Check sheet for the modelled part. Datum: model origin and axes. Units: mm. Round coordinates to 2 decimals unless told otherwise and drop trailing zeros. Write each loop counter-clockwise with the first axis right and the second up, starting at its lowest first coordinate (ties: lowest second). Pieces come first, ordered by that corner, then holes. Notation, with made-up numbers: (10.25, 19.5) -> (17.25, 19.5) arc R14 cw to (17.25, 41.5) -> close; hole circle Ø7 at (56.5, 8). An arc over 180 degrees is marked (long way). One line per item, written item: value.
from build123d import *

# Parameters (mm, degrees)
F1_DEPTH = 10
F3_DEPTH = 35
F5_DEPTH = 45.001


with BuildPart() as f1:
    # F0 (on Right) → F1 (new body)
    with BuildSketch(Plane.YZ):
        with BuildLine():
            ThreePointArc((0, 0), (-34.0398401022, -11.614694955), (-68.0796802044, 0))
            ThreePointArc((-68.0796802044, 0), (-43.0772294723, -14.2909034111), (-14.4906720078, -10.8036128804))
            ThreePointArc((-14.4906720078, -10.8036128804), (-6.7062533875, -6.1248672779), (0, 0))
        make_face()
        with BuildLine():
            ThreePointArc((0, 0), (-6.7062533875, -6.1248672779), (-14.4906720078, -10.8036128804))
            Line((-14.4906720078, -10.8036128804), (0, -10.8036128804))
            Line((0, -10.8036128804), (0, 0))
        make_face()
    extrude(amount=F1_DEPTH)

    # F2 (on face) → F3 (join)
    with BuildSketch(Plane(origin=(0, 0, 0), x_dir=(0, -1, 0), z_dir=(-1, 0, 0))):
        with BuildLine():
            Line((0, -10.8036128804), (14.4906720078, -10.8036128804))
            Line((14.4906720078, -10.8036128804), (14.4906720078, -8.0706065552))
            ThreePointArc((14.4906720078, -8.0706065552), (6.9431775325, -4.5778249918), (0, 0))
            Line((0, 0), (0, -10.8036128804))
        make_face()
    extrude(amount=F3_DEPTH)

    # F4 (on face) → F5 (cut, through all)
    with BuildSketch(Plane.YZ.offset(10)):
        with BuildLine():
            Line((-14.4906720078, -8.0706065552), (-14.4906720078, -10.8036128804))
            Line((-14.4906720078, -10.8036128804), (0, -10.8036128804))
            Line((0, -10.8036128804), (0, 0))
            ThreePointArc((0, 0), (-6.9431775325, -4.5778249918), (-14.4906720078, -8.0706065552))
        make_face()
    extrude(amount=-F5_DEPTH, mode=Mode.SUBTRACT)


solid = f1.part
Item 1: Sectioned sample at A-A (z = -8.75). Enter the section's corners in (x, y), then the cut area to 3 significant figures.
Result set:
outline: (0, -57.44) -> (10, -57.44) -> (10, -51.67) -> (0, -51.67) -> close; (0, -16.41) -> (10, -16.41) -> (10, -14.49) -> (0, -14.49) -> close
area: 76.9 mm^2
Item 2: Sectioned sample at C-C (y = -19.5). Enter the section's corners in (x, z), then the cut area to 3 significant figures.
Result set:
outline: (0, -12.82) -> (10, -12.82) -> (10, -9.68) -> (0, -9.68) -> close
area: 31.4 mm^2
Item 3: Sectioned sample at B-B (x = 8). Enter the section's corners in (y, z).
Result set:
outline: (-68.08, 0) arc R45.73 ccw to (-14.49, -10.8) -> (-14.49, -8.07) arc R55.69 cw to start
Item 4: Depth check by flat-ended pin: pin 1 (2 mm diameter, centred on x = 3, y = -48, fed in from -Z); pin 2 (6 mm diameter, centred on x = 3.5, z = -3.5, fed in from +Y). Enter the tip coordinate at first touch or a pass-through.
Result set:
pin 1: z = -13.32
pin 2: y = -57.35
Item 5: Sectioned sample at D-D (z = -5.5). Enter the section's corners in (x, y), then the cut area to 3 significant figures.
Result set:
outline: (0, -62.19) -> (10, -62.19) -> (10, -59.41) -> (0, -59.41) -> close
area: 27.8 mm^2
Item 6: Material ranges on line 1 along Z through (x, y) = (2, -23); line 2 along Z through (x, y) = (5.25, -25); line 3 along Y through (x, z) = (4.75, -1), recorded low to high.
Result set:
line 1: -13.84 to -10.51
line 2: -14.29 to -10.88
line 3: -67.16 to -66.74
